Read the model definition and answer for the solid it produces. Units are mm, in the model's axes. Round coordinates to 2 decimals unless told otherwise and drop trailing zeros. Loops run counter-clockwise (first coordinate to the right, second up) from the corner with the lowest first, then second, coordinate; pieces in that order, holes last. Notation, with made-up numbers: (76.5, 65) - (105.5, 65) arc R15 cw to (105.5, 71) - close; hole circle Ø8 at (1.5, -36.75). An arc over 180 degrees is marked (long way). Answer as CSV lines item,"result".
```python
from build123d import *

# Parameters (mm, degrees)
REVOLVE3_ANGLE     = 180
CUT_EXTRUDE2_DEPTH = 6.985


with BuildPart() as part:
    # Sketch1 → Revolve3 (revolve)
    with BuildSketch(Plane.XY):
        with BuildLine():
            Line((-57.135887146, 44.45), (-35.56, 44.45))
            Line((-35.56, 44.45), (-35.56, 57.15))
            Line((-35.56, 57.15), (0, 57.15))
            Line((0, 57.15), (0, 72.39))
            Line((0, 72.39), (0, 80.01))
            ThreePointArc((0, 80.01), (-37.717075708, 70.562187466), (-66.526668337, 44.45))
            Line((-66.526668337, 44.45), (-57.135887146, 44.45))
        make_face()
    revolve3 = revolve(axis=Axis((0, 57.15, 0), (0, 1, 0)), revolution_arc=REVOLVE3_ANGLE)

    # Sketch4 → Cut-Extrude2 (cut)
    with BuildSketch(Plane(origin=(0, 0, 0), x_dir=(-1, 0, 0), z_dir=(0, 0, -1))):
        with BuildLine():
            Line((-66.526668337, 44.45), (-57.135887146, 44.45))
            ThreePointArc((-57.135887146, 44.45), (0, 72.39), (57.135887146, 44.45))
            Line((57.135887146, 44.45), (66.526668337, 44.45))
            ThreePointArc((66.526668337, 44.45), (0, 80.01), (-66.526668337, 44.45))
        make_face()
    cut_extrude2 = extrude(amount=-CUT_EXTRUDE2_DEPTH, mode=Mode.SUBTRACT)

    # Mirror1: Revolve3, Cut-Extrude2 across Front Plane
    add(revolve3.mirror(Plane.XY))
    add(cut_extrude2.mirror(Plane.XY), mode=Mode.SUBTRACT)


solid = part.part
```
1) A cutting plane is placed at A-A, the plane x = 0. Determine the outline of the cut face in (y, z) (3 decimals).
Entries:
outline,"(44.45, -66.527) arc R80.01 ccw to (79.705, -6.985) - (72.39, -6.985) - (72.39, 6.985) - (79.705, 6.985) arc R80.01 ccw to (44.45, 66.527) - (44.45, 35.56) - (57.15, 35.56) - (57.15, -35.56) - (44.45, -35.56) - close"
2) A cutting plane is placed at C-C, the plane y = 69.5. Determine the outline of the cut face in (x, z) (3 decimals), plus the area to 3 significant figures.
Entries:
outline,"(-39.02, -6.985) arc R39.64 ccw to (39.02, -6.985) - (20.25, -6.985) - (20.25, 6.985) - (39.02, 6.985) arc R39.64 ccw to (-39.02, 6.985) - (-20.25, 6.985) - (-20.25, -6.985) - close"
area,"4,400 mm^2"
3) Find the intervals of material crossed by line 1 (Z direction, x = 31.5, y = 50.5); line 2 (X direction, y = 57, z = -9); line 3 (Z direction, x = 12, y = 51.5), in increasing order.
Entries:
line 1,"z = -53.47 to -16.5, 16.5 to 53.47"
line 2,"x = -55.42 to -34.4, 34.4 to 55.42"
line 3,"z = -60.04 to -33.47, 33.47 to 60.04"
4) Each of these flat-tipped pins is pushed along its axis until it touches: P1, Ø6, axis at x = 52, z = 29, coming from the +Y side; P2, Ø17.5, axis at x = -6, y = 64.5, coming from the +Z side; P3, Ø1, axis at y = 63, z = -27.5, coming from the +X side; P4, Ø8, axis at x = 47.5, y = 73, coming from the +Z side. Where does it stop, or does it pass through?
Entries:
P1,"stops at y = 56.61"
P2,"stops at z = 57.12"
P3,"stops at x = 41.77"
P4,"passes through"
5) A cutting plane is placed at D-D, the plane z = 4. Determine the outline of the cut face in (x, y).
Entries:
outline,"(-57.14, 44.45) - (-35.33, 44.45) - (-35.33, 57.15) - (35.33, 57.15) - (35.33, 44.45) - (57.14, 44.45) arc R72.39 ccw to start"
6) A cutting plane is placed at B-B, the plane y = 49. Determine the outline of the cut face in (x, z) (3 decimals), plus the area to 3 significant figures.
Entries:
outline,"(-62.863, -6.985) arc R63.25 ccw to (62.863, -6.985) - (53.285, -6.985) - (53.285, 6.985) - (62.863, 6.985) arc R63.25 ccw to (-62.863, 6.985) - (-53.285, 6.985) - (-53.285, -6.985) - close; hole circle Ø71.12 at (0, 0)"
area,"8,320 mm^2"
